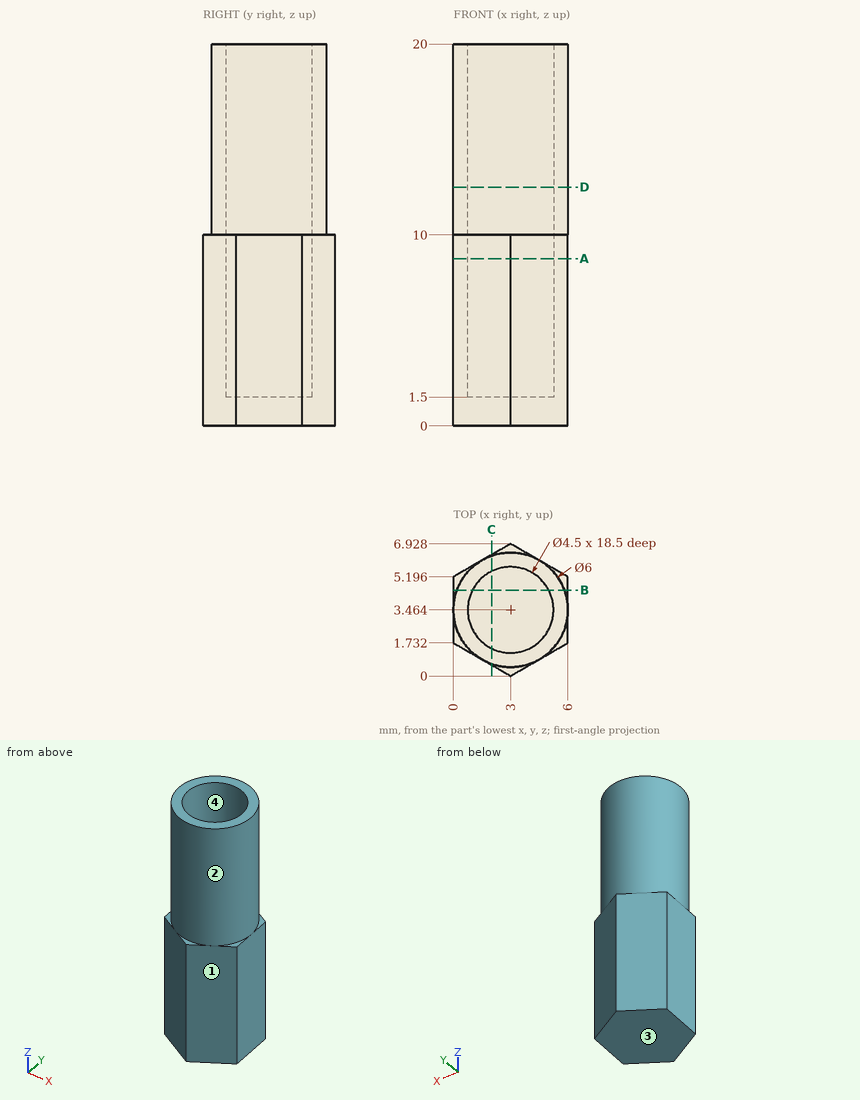
The drawing under review shows one solid part. Ordinate dimensions are in mm from its lowest x, y, z. Round coordinates to 2 decimals unless told otherwise and drop trailing zeros. Write each loop counter-clockwise with the first axis right and the second up, starting at its lowest first coordinate (ties: lowest second). Pieces come first, ordered by that corner, then holes. Notation, with made-up numbers: (83.25, 1.5) - (115.25, 1.5) arc R10 cw to (115.25, 6.5) - close; hole circle Ø8 at (10, -30.75). An arc over 180 degrees is marked (long way). Use a Markdown table: item, result. Add a question column.
1. We need section A-A (z = 8.75). State the section outline as (x, y) points, then the cut area to 3 significant figures.
2. Wall thickness on probe 1 along Y at (x, z) = (3, 15.25); probe 2 along Y at (x, z) = (2.25, 11.25) (1 decimal); probe 3 along Z at (x, y) = (1, 4.25): over which ranges is each line inside the solid? List them lowest first.
3. We need section B-B (y = 4.5). State the section outline as (x, z) points, then the cut area to 3 significant figures.
4. Mouldability with a two-part tool opening along Y and no side actions: class the marked faces 1, 2, 3 and 4 as +Y half, -Y half, draft (parallel to the pull), parting line (faces both ways), or undercut.
5. We need section D-D (z = 12.5). State the section outline as (x, y) points, then the cut area to 3 significant figures.
6. Clearance check with a flat-ended pin moving along its axis: pin 1 (1 mm diameter, centred on x = 2.5, y = 4.5, fed in from +Z). State where the tip first meets the part, or that it passes through.
7. We need section C-C (x = 2). State the section outline as (y, z) points.
Output:
| question | item | result |
|---|---|---|
| 1 | outline | (0, 1.73) - (3, 0) - (6, 1.73) - (6, 5.2) - (3, 6.93) - (0, 5.2) - close; hole circle Ø4.5 at (3, 3.46) |
| 1 | area | 15.3 mm2 |
| 2 | probe 1 | y = 0.46 to 1.21, 5.71 to 6.46 |
| 2 | probe 2 | y = 0.6 to 1.3, 5.6 to 6.4 |
| 2 | probe 3 | z = 0 to 1.5 |
| 3 | outline | (0, 0) - (6, 0) - (6, 10) - (5.82, 10) - (5.82, 20) - (5, 20) - (5, 1.5) - (1, 1.5) - (1, 20) - (0.18, 20) - (0.18, 10) - (0, 10) - close |
| 3 | area | 42.4 mm2 |
| 4 | face 1 | -Y half |
| 4 | face 2 | parting line |
| 4 | face 3 | draft |
| 4 | face 4 | undercut |
| 5 | outline | circle Ø6 at (3, 3.46); hole circle Ø4.5 at (3, 3.46) |
| 5 | area | 12.4 mm2 |
| 6 | pin 1 | stops at z = 1.5 |
| 7 | outline | (0.58, 0) - (6.35, 0) - (6.35, 10) - (6.29, 10) - (6.29, 20) - (5.48, 20) - (5.48, 1.5) - (1.45, 1.5) - (1.45, 20) - (0.64, 20) - (0.64, 10) - (0.58, 10) - close |
